```python
from build123d import *

# Parameters (mm, degrees)
SKETCH_1_R               = 45
SKETCH_1_R_2             = 37
SKETCH_1_R_3             = 1.7
EXTRUDE_1_DEPTH          = 10.5
CUT_EXTRUDE_START        = -3
CUT_EXTRUDE_1_DEPTH      = 3
PATTERN_CIRCULAR_1_COUNT = 4
CUT_EXTRUDE_START_2      = -13
CUT_EXTRUDE_2_DEPTH      = 13


with BuildPart() as part:
    # 草图1 → 凸台-拉伸1 (new body)
    with BuildSketch(Plane.XY):
        with Locations(Location((0, 0, 0), (0, 0, 180))):
            Circle(SKETCH_1_R)
        with Locations(Location((0, 0, 0), (0, 0, 180))):
            Circle(SKETCH_1_R_2, mode=Mode.SUBTRACT)
        with Locations(Location((41, 0, 0), (0, 0, 180))):
            Circle(SKETCH_1_R_3, mode=Mode.SUBTRACT)
        with Locations(Location((0, -41, 0), (0, 0, 180))):
            Circle(SKETCH_1_R_3, mode=Mode.SUBTRACT)
        with Locations(Location((-41, 0, 0), (0, 0, 180))):
            Circle(SKETCH_1_R_3, mode=Mode.SUBTRACT)
        with Locations(Location((0, 41, 0), (0, 0, 180))):
            Circle(SKETCH_1_R_3, mode=Mode.SUBTRACT)
    extrude(amount=EXTRUDE_1_DEPTH)

    # 草图2 → 切除-拉伸1 (cut)
    with BuildSketch(Plane.XY.offset(10.5).offset(CUT_EXTRUDE_START)):
        with BuildLine():
            Line((9.356026087, 44.016642033), (7.69273256, 36.191461227))
            ThreePointArc((7.69273256, 36.191461227), (26.162950904, 26.162950904), (36.191461227, 7.69273256))
            Line((36.191461227, 7.69273256), (44.016642033, 9.356026087))
            ThreePointArc((44.016642033, 9.356026087), (31.819805153, 31.819805153), (9.356026087, 44.016642033))
        make_face()
    cut_extrude_1 = extrude(amount=CUT_EXTRUDE_1_DEPTH, mode=Mode.SUBTRACT)

    # 阵列(圆周)1: 切除-拉伸1 ×4 about axis
    pattern_circular_1_axis = Axis((0, 0, 10.5), (0, 0, -1))
    for i in range(1, PATTERN_CIRCULAR_1_COUNT):
        add(cut_extrude_1.rotate(pattern_circular_1_axis, i * 360 / PATTERN_CIRCULAR_1_COUNT), mode=Mode.SUBTRACT)

    # 草图3 → 切除-拉伸2 (cut)
    with BuildSketch(Plane.XY.offset(7.5).offset(CUT_EXTRUDE_START_2)):
        with BuildLine():
            Line((34.768626969, -12.654745303), (42.286167935, -15.39090645))
            ThreePointArc((42.286167935, -15.39090645), (31.819805153, -31.819805153), (15.39090645, -42.286167935))
            Line((15.39090645, -42.286167935), (12.654745303, -34.768626969))
            ThreePointArc((12.654745303, -34.768626969), (26.162950904, -26.162950904), (34.768626969, -12.654745303))
        make_face()
    extrude(amount=CUT_EXTRUDE_2_DEPTH, mode=Mode.SUBTRACT)


solid = part.part
```
For this review, take the finished solid that the model builds, in its own axes (mm). A direction names the side the tool comes from. Round coordinates to 2 decimals unless told otherwise and drop trailing zeros. Write each loop counter-clockwise with the first axis right and the second up, starting at its lowest first coordinate (ties: lowest second). Pieces come first, ordered by that corner, then holes. Notation, with made-up numbers: (-13, 0.25) - (34, 0.25) arc R22 cw to (34, 29.25) - close; hole circle Ø3 at (-29.75, 62.5). An arc over 180 degrees is marked (long way). Answer as CSV lines item,"result". Start each with the question number.
(1) For pin 1 (4 mm diameter, centred on x = 15.5, z = 5.5, fed in from -Y); pin 2 (11 mm diameter, centred on x = 27.5, y = 19.5, fed in from +Z); pin 3 (2.5 mm diameter, centred on x = 41, y = 0, fed in from -Z); pin 4 (6 mm diameter, centred on x = 24, z = 4, fed in from -Y), all flat-tipped, find the tip position at first contact; note any pin that passes through.
(2) For line 1 (Y direction, x = 0, z = 7); line 2 (Y direction, x = -1.5, z = 7.5) (3 decimals); line 3 (Z direction, x = 14, y = 35.5), list the stretches that pass through material, from the lowest coordinate up.
(3) Add section C-C, the plane x = -30. State the section outline as (y, z) points.
(4) Mouldability with a two-part tool opening along Y and no side actions: class faces 1 (the flat face through (40.049, 8.513, 8.979)), 2 (the cylindrical face through (42.35, 1.03, 5.18)), 3 (the cylindrical face through (-30.592, 33.002, 4.01)), 4 (the flat face through (8.513, -40.049, 8.979)) as +Y half, -Y half, draft (parallel to the pull), parting line (faces both ways), or undercut.
(5) Add section A-A, the plane y = 0. State the section outline as (x, z) points.
(6) Add section B-B, the plane z = 3.5. State the section outline as (x, y) points, plus the area to 3 significant figures.
(7) Add section D-D, the plane y = -41. State the section outline as (x, z) points.
(8) Machinability: for faces 5 (the flat face through (40.159, -8.536, 8.979)), 6 (the flat face through (-8.513, 40.049, 8.979)), 7 (the flat face through (12, -39, 7.5)), which of the approach directions +Z, -Z, +X, -X, +Y, -Y give a long, thin tool a straight path to every point of the face, cutting with its end or side? Answer none if there is none.
From the geometry:
1,pin 1,"stops at y = -42.93"
1,pin 2,"stops at z = 7.5"
1,pin 3,"passes through"
1,pin 4,"stops at y = 25.3"
2,line 1,"y = -45 to -42.7, -39.3 to -37, 37 to 39.3, 42.7 to 45"
2,line 2,"y = -44.975 to -41.8, -40.2 to -36.97, 36.97 to 40.2, 41.8 to 44.975"
2,line 3,"z = 0 to 7.5"
3,outline,"(-33.54, 0) - (-21.66, 0) - (-21.66, 7.5) - (-33.54, 7.5) - close; (21.66, 0) - (33.54, 0) - (33.54, 7.5) - (21.66, 7.5) - close"
4,face 1,"+Y half"
4,face 2,"undercut"
4,face 3,"parting line"
4,face 4,"undercut"
5,outline,"(-45, 0) - (-42.7, 0) - (-42.7, 10.5) - (-45, 10.5) - close; (-39.3, 0) - (-37, 0) - (-37, 10.5) - (-39.3, 10.5) - close; (37, 0) - (39.3, 0) - (39.3, 10.5) - (37, 10.5) - close; (42.7, 0) - (45, 0) - (45, 10.5) - (42.7, 10.5) - close"
6,outline,"(12.65, -34.77) arc R37 cw (long way) to (34.77, -12.65) - (42.29, -15.39) arc R45 ccw (long way) to (15.39, -42.29) - close; hole circle Ø3.4 at (-41, 0); hole circle Ø3.4 at (0, -41); hole circle Ø3.4 at (0, 41); hole circle Ø3.4 at (41, 0)"
6,area,"1,740 mm²"
7,outline,"(-18.55, 0) - (-1.7, 0) - (-1.7, 10.5) - (-8.71, 10.5) - (-8.71, 7.5) - (-18.55, 7.5) - close; (1.7, 0) - (14.92, 0) - (14.92, 7.5) - (8.71, 7.5) - (8.71, 10.5) - (1.7, 10.5) - close"
8,face 5,"+Z, -Y"
8,face 6,"+Z, -X"
8,face 7,"+Z, +X"
